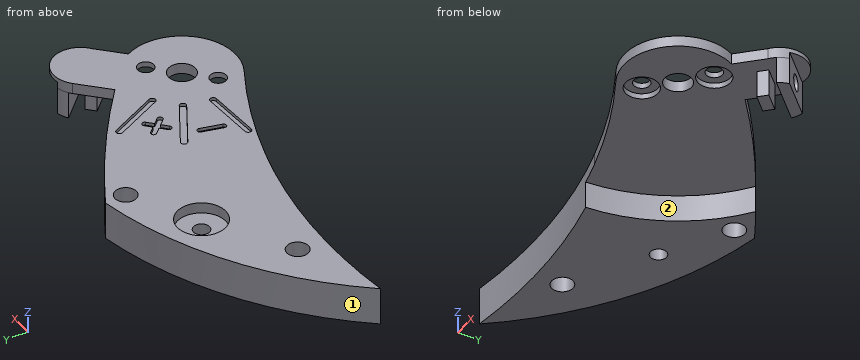
from build123d import *

# Parameters (mm, degrees)
CROQUIS1_R                 = 0.625
CROQUIS1_R_2               = 0.5
SALIENTE_EXTRUIR1_DEPTH    = 1.75
CROQUIS2_R                 = 7.75
CORTAR_EXTRUIR1_DEPTH      = 1.25
SALIENTE_EXTRUIR2_DEPTH    = 1.25
CORTAR_EXTRUIR2_DEPTH      = 0.3
CROQUIS5_R                 = 0.75
CORTAR_EXTRUIR3_DEPTH      = 0.25
CROQUIS7_R                 = 1.125
CORTAR_EXTRUIR4_DEPTH      = 0.5
CORTAR_EXTRUIR5_DEPTH      = 0.15
M1X0_25_TAPPED_HOLE1_D     = 0.75
M1X0_25_TAPPED_HOLE2_D     = 0.75
M1X0_25_TAPPED_HOLE3_D     = 0.75
M1X0_25_TAPPED_HOLE3_DEPTH = 0.5


with BuildPart() as part:
    # Croquis1 → Saliente-Extruir1 (new body)
    with BuildSketch(Plane.XY):
        with BuildLine():
            Line((6.259644122, 12.249974926), (5.198983951, 11.189314754))
            ThreePointArc((5.198983951, 11.189314754), (4.763256008, 8.227733584), (1.799492386, 7.807106599))
            ThreePointArc((1.799492386, 7.807106599), (-0.79068784, 9.047504388), (-3.5, 10))
            ThreePointArc((-3.5, 10), (-8.600559157, 10.927738054), (-13.78279853, 10.783527469))
            ThreePointArc((-13.78279853, 10.783527469), (-9.016404165, 14.998481788), (-3.058096956, 17.230729613))
            ThreePointArc((-3.058096956, 17.230729613), (0.268930152, 15.227921239), (3.386067713, 12.911932422))
            Line((3.386067713, 12.911932422), (4.62350458, 14.14936929))
            ThreePointArc((4.62350458, 14.14936929), (6.451492666, 14.069616403), (6.259644122, 12.249974926))
        make_face()
        with Locations((3, 10)):
            Circle(CROQUIS1_R, mode=Mode.SUBTRACT)
        with Locations((-3, 16.25)):
            Circle(CROQUIS1_R_2, mode=Mode.SUBTRACT)
        with Locations((-9.75, 12.25)):
            Circle(CROQUIS1_R_2, mode=Mode.SUBTRACT)
    extrude(amount=SALIENTE_EXTRUIR1_DEPTH)

    # Croquis2 → Cortar-Extruir1 (cut)
    with BuildSketch(Plane(origin=(0, 0, 0), x_dir=(-1, 0, 0), z_dir=(0, 0, -1))):
        with Locations((-3, 10)):
            Circle(CROQUIS2_R)
    extrude(amount=-CORTAR_EXTRUIR1_DEPTH, mode=Mode.SUBTRACT)

    # Croquis3 → Saliente-Extruir2 (add)
    with BuildSketch(Plane(origin=(0, 0, 1.25), x_dir=(-1, 0, 0), z_dir=(0, 0, -1))):
        Polygon((-5.272601551, 12.323592527), (-4.56549477, 13.030699308), (-4.91904816, 13.384252698), (-5.626154942, 12.677145917), align=None)
        with BuildLine():
            Line((-6.508612401, 12.501795239), (-4.751795239, 14.258612401))
            ThreePointArc((-4.751795239, 14.258612401), (-4.983609366, 14.394748904), (-5.239087061, 14.47842736))
            Line((-5.239087061, 14.47842736), (-6.72842736, 12.989087061))
            ThreePointArc((-6.72842736, 12.989087061), (-6.644748904, 12.733609366), (-6.508612401, 12.501795239))
        make_face()
    extrude(amount=SALIENTE_EXTRUIR2_DEPTH)

    # Croquis4 → Cortar-Extruir2 (cut)
    with BuildSketch(Plane(origin=(0, 0, 1.25), x_dir=(-1, 0, 0), z_dir=(0, 0, -1))):
        with BuildLine():
            Line((-5.239087061, 14.47842736), (-6.72842736, 12.989087061))
            ThreePointArc((-6.72842736, 12.989087061), (-6.388006008, 14.138006008), (-5.239087061, 14.47842736))
        make_face()
    extrude(amount=-CORTAR_EXTRUIR2_DEPTH, mode=Mode.SUBTRACT)

    # Croquis5 → Cortar-Extruir3 (cut)
    with BuildSketch(Plane(origin=(0, 0, 1.25), x_dir=(-1, 0, 0), z_dir=(0, 0, -1))):
        with Locations((-4.060660172, 11.060660172)):
            Circle(CROQUIS5_R)
        with Locations((-1.939339828, 8.939339828)):
            Circle(CROQUIS5_R)
    extrude(amount=-CORTAR_EXTRUIR3_DEPTH, mode=Mode.SUBTRACT)

    # Croquis7 → Cortar-Extruir4 (cut)
    with BuildSketch(Plane.XY.offset(1.75)):
        with Locations((-6, 14.5)):
            Circle(CROQUIS7_R)
    extrude(amount=-CORTAR_EXTRUIR4_DEPTH, mode=Mode.SUBTRACT)

    # Croquis8 → Cortar-Extruir5 (cut)
    with BuildSketch(Plane.XY.offset(1.75)):
        with BuildLine():
            Line((0.977196105, 14.300379565), (2.112172354, 12.072863254))
            ThreePointArc((2.112172354, 12.072863254), (2.046619951, 11.871113701), (1.844870397, 11.936666104))
            Line((1.844870397, 11.936666104), (0.709894148, 14.164182415))
            ThreePointArc((0.709894148, 14.164182415), (0.775446551, 14.365931969), (0.977196105, 14.300379565))
        make_face()
        with BuildLine():
            Line((0.76093394, 9.732449668), (-1.735639897, 9.601609778))
            ThreePointArc((-1.735639897, 9.601609778), (-1.89328472, 9.743553814), (-1.751340684, 9.901198638))
            Line((-1.751340684, 9.901198638), (0.745233153, 10.032038529))
            ThreePointArc((0.745233153, 10.032038529), (0.902877977, 9.890094492), (0.76093394, 9.732449668))
        make_face()
        with BuildLine():
            Line((-1.038620668, 12.504903811), (1.126442841, 11.254903811))
            ThreePointArc((1.126442841, 11.254903811), (1.181346652, 11.05), (0.976442841, 10.995096189))
            Line((0.976442841, 10.995096189), (-1.188620668, 12.245096189))
            ThreePointArc((-1.188620668, 12.245096189), (-1.243524479, 12.45), (-1.038620668, 12.504903811))
        make_face()
        with BuildLine():
            Line((-0.633682247, 11.386577522), (-0.867127611, 10.414207601))
            ThreePointArc((-0.867127611, 10.414207601), (-1.017854522, 10.321842032), (-1.110220091, 10.472568942))
            Line((-1.110220091, 10.472568942), (-0.876774727, 11.444938863))
            ThreePointArc((-0.876774727, 11.444938863), (-0.726047817, 11.537304432), (-0.633682247, 11.386577522))
        make_face()
        with BuildLine():
            Line((-0.053831977, 12.491697608), (0.218183412, 12.749830574))
            Line((0.218183412, 12.749830574), (-0.039949554, 13.021845963))
            ThreePointArc((-0.039949554, 13.021845963), (-0.03532208, 13.198562081), (0.141394039, 13.193934607))
            Line((0.141394039, 13.193934607), (0.399527005, 12.921919218))
            Line((0.399527005, 12.921919218), (0.671542394, 13.180052184))
            ThreePointArc((0.671542394, 13.180052184), (0.848258512, 13.175424709), (0.843631038, 12.998708591))
            Line((0.843631038, 12.998708591), (0.571615649, 12.740575625))
            Line((0.571615649, 12.740575625), (0.829748614, 12.468560236))
            ThreePointArc((0.829748614, 12.468560236), (0.82512114, 12.291844118), (0.648405022, 12.296471592))
            Line((0.648405022, 12.296471592), (0.390272056, 12.568486981))
            Line((0.390272056, 12.568486981), (0.118256667, 12.310354015))
            ThreePointArc((0.118256667, 12.310354015), (-0.058459452, 12.31498149), (-0.053831977, 12.491697608))
        make_face()
    extrude(amount=-CORTAR_EXTRUIR5_DEPTH, mode=Mode.SUBTRACT)

    # M1x0.25 Tapped Hole1 (through all)
    with Locations(Plane(origin=(0, 0, 1.5), x_dir=(-1, 0, 0), z_dir=(0, 0, -1))):
        with Locations((-1.939339828, 8.939339828), (-4.060660172, 11.060660172)):
            Hole(M1X0_25_TAPPED_HOLE1_D / 2)

    # M1x0.25 Tapped Hole2 (through all)
    with Locations(Plane.XY.offset(1.25)):
        with Locations((-6, 14.5)):
            Hole(M1X0_25_TAPPED_HOLE2_D / 2)

    # M1x0.25 Tapped Hole3
    with Locations(Plane(origin=(9.858757211, 9.858757211, 0), x_dir=(-0.707106781, 0.707106781, 0), z_dir=(0.707106781, 0.707106781, 0))):
        with Locations((5.480077554, 0.775)):
            Hole(M1X0_25_TAPPED_HOLE3_D / 2, depth=M1X0_25_TAPPED_HOLE3_DEPTH)


solid = part.part
Geometry check sheet. Reference: the model listing, model coordinates, mm. Face numbers are marked on the shaded views. A direction names the side the tool comes from. Coordinates: 2 decimals unless noted, no trailing zeros. Write each loop counter-clockwise with the first axis right and the second up, starting at its lowest first coordinate (ties: lowest second). Pieces come first, ordered by that corner, then holes. Notation, with made-up numbers: (71.25, 30.25) -> (87.25, 30.25) arc R15 ccw to (87.25, 38.25) -> close; hole circle Ø3 at (0.25, -7). An arc over 180 degrees is marked (long way). One line per question, with ' | ' between items.
1. Cross-section at A-A on x = -9.75. Record the cut outline in (y, z).
Answers:
outline: (10.99, 0) -> (11.75, 0) -> (11.75, 1.75) -> (10.99, 1.75) -> close; (12.75, 0) -> (14.53, 0) -> (14.53, 1.75) -> (12.75, 1.75) -> close
2. Set-up check for the marked faces 1 and 2: record each of +Z, -Z, +X, -X, +Y, -Y from which the full face is reachable in a straight line by a thin tool's end or side.
Answers:
face 1: +Z, -Z, -X, +Y | face 2: -Z, -Y
3. Depth check by flat-ended pin: pin 1 Ø1.6 at (x, y) = (4, 11.5) entering from -Z; pin 2 Ø0.5 at (x, y) = (6.5, 13.5) entering from -Z; pin 3 Ø1 at (x, z) = (-10.5, 0.5) entering from +Y; pin 4 Ø2 at (x, y) = (-6, 14.5) entering from +Z. Enter the tip coordinate at first touch or a pass-through.
Answers:
pin 1: stops at z = 1.25 | pin 2: stops at z = 0 | pin 3: stops at y = 14.36 | pin 4: stops at z = 1.25
4. Cross-section at B-B on x = -6. Record the cut outline in (y, z) (3 decimals).
Answers:
outline: (10.592, 0) -> (14.125, 0) -> (14.125, 1.25) -> (13.375, 1.25) -> (13.375, 1.75) -> (10.592, 1.75) -> close; (14.875, 0) -> (16.439, 0) -> (16.439, 1.75) -> (15.625, 1.75) -> (15.625, 1.25) -> (14.875, 1.25) -> close
5. Thickness scan on probe 1 along Z at (x, y) = (-2, 10.75); probe 2 along X at (y, z) = (14.25, 1.45); probe 3 along X at (y, z) = (13.25, 0.1). Record the ranges inside material, lowest first. Write a range as from..to.
Answers:
probe 1: z = 1.25..1.75 | probe 2: x = -10.16..-7.1, -4.9..1.66, 4.74..5.47 | probe 3: x = -11.43..-4.04, 4.78..5.05, 5.76..6.47
